```python
from build123d import *

# Parameters (mm, degrees)
F0_W      = 1120
F0_H      = 722
F1_DEPTH  = 40
F2_W      = 70
F2_H      = 725
F3_DEPTH  = 10
F5_D      = 30
F7_D      = 30
F8_W      = 70
F8_H      = 725
F9_DEPTH  = 10
F11_D     = 30
F12_W     = 1060
F12_H     = 680
F13_DEPTH = 40.001


with BuildPart() as f1:
    # F0 (on Front) → F1 (new body)
    with BuildSketch(Plane.XZ):
        Rectangle(F0_W, F0_H)
    extrude(amount=F1_DEPTH)

    # F2 (on Front) → F3 (join)
    with BuildSketch(Plane.XZ):
        with Locations((590, 0)):
            Rectangle(F2_W, F2_H)
    extrude(amount=F3_DEPTH)

    # F5 (through all)
    with Locations(Plane.XZ.offset(10)):
        with Locations((585, 142.5)):
            Hole(F5_D / 2)

    # F7 (through all)
    with Locations(Plane.XZ.offset(10)):
        with Locations((585, -142.5)):
            Hole(F7_D / 2)

    # F8 (on Front) → F9 (join)
    with BuildSketch(Plane.XZ):
        with Locations((-590, 0)):
            Rectangle(F8_W, F8_H)
    extrude(amount=F9_DEPTH)

    # F11 (through all)
    with Locations(Plane.XZ.offset(10)):
        with Locations((-585, 142.5), (-585, -142.556826)):
            Hole(F11_D / 2)

    # F12 (on face) → F13 (cut, through all)
    with BuildSketch(Plane.XZ.offset(40)):
        Rectangle(F12_W, F12_H)
    extrude(amount=-F13_DEPTH, mode=Mode.SUBTRACT)


solid = f1.part
```
Work out the finished part from the listing and answer in its coordinate system (mm). A direction names the side the tool comes from. Give positions to 0.01 mm unless a question says otherwise; leave off trailing zeros. Order: outer loops, then holes, each group sorted by start corner. A loop starts at its lowest first (then second) coordinate and runs counter-clockwise, first axis right, second up. Notation, with made-up numbers: (45, 45) -> (85, 45) arc R21 ccw to (85, 77) -> close; hole circle Ø6 at (31, 19). An arc over 180 degrees is marked (long way). Answer as CSV lines item,"result". Start each with the question number.
(1) Section D-D, the plane y = -27 is taken. Write down the section's boundary in (x, z).
(2) For a pull along Z with two mould halves and no side action, classify faces 4 (the flat face through (560, -25, -5)), 5 (the cylindrical face through (596.9, -4.93, 133.37)), 6 (the flat face through (-7, -20, -340)) as released by +Z, released by -Z, zero draft, split by the parting line, or undercut.
(3) Each of these flat-tipped pins is pushed along its axis until it touches: pin 1 Ø1.5 at (x, y) = (293.5, -9) entering from +Z; pin 2 Ø20 at (x, y) = (41.5, -10.5) entering from -Z; pin 3 Ø18 at (x, z) = (-585, 142.5) entering from -Y; pin 4 Ø8 at (y, z) = (-30.5, -220) entering from -X. Where does it stop, or does it pass through?
(4) Section C-C, the plane x = 585 is taken. Write down the section's boundary in (y, z), plus the area to 3 significant figures.
(5) Consider line 1 along Z through (x, y) = (585, -3.25); line 2 along X through (y, z) = (-31.5, 123); line 3 along Z through (x, y) = (-585, -2). Determine where each line is inside the solid, lowest interval first.
(6) Section A-A, the plane z = -276.5 is taken. Write down the section's boundary in (x, y).
(7) Which of the six approach directions +Z, -Z, +X, -X, +Y, -Y give full straight-line access (tool end or side, diameter ignored) to faces 1 (the flat face through (-560, -25, -5)), 2 (the flat face through (-7, -20, 340)), 3 (the flat face through (-3, 0, 351))?
(8) Section B-B, the plane z = 142.5 is taken. Write down the section's boundary in (x, y).
Entries:
1,outline,"(-560, -361) -> (560, -361) -> (560, 361) -> (-560, 361) -> close; hole (-530, -340) -> (530, -340) -> (530, 340) -> (-530, 340) -> close"
2,face 4,"zero draft"
2,face 5,"undercut"
2,face 6,"undercut"
3,pin 1,"z = 361"
3,pin 2,"z = -361"
3,pin 3,"through"
3,pin 4,"x = -560"
4,outline,"(-10, -362.5) -> (0, -362.5) -> (0, -157.5) -> (-10, -157.5) -> close; (-10, -127.5) -> (0, -127.5) -> (0, 127.5) -> (-10, 127.5) -> close; (-10, 157.5) -> (0, 157.5) -> (0, 362.5) -> (-10, 362.5) -> close"
4,area,"6,650 mm²"
5,line 1,"-362.5 to -157.5, -127.5 to 127.5, 157.5 to 362.5"
5,line 2,"-560 to -530, 530 to 560"
5,line 3,"-362.5 to -157.56, -127.56 to 127.5, 157.5 to 362.5"
6,outline,"(-625, -10) -> (-560, -10) -> (-560, -40) -> (-530, -40) -> (-530, 0) -> (-625, 0) -> close; (530, -40) -> (560, -40) -> (560, -10) -> (625, -10) -> (625, 0) -> (530, 0) -> close"
7,face 1,"+Z, -Z, -X, -Y"
7,face 2,"+Y, -Y"
7,face 3,"+Z, -Z, +X, -X, +Y"
8,outline,"(-625, -10) -> (-600, -10) -> (-600, 0) -> (-625, 0) -> close; (-570, -10) -> (-560, -10) -> (-560, -40) -> (-530, -40) -> (-530, 0) -> (-570, 0) -> close; (530, -40) -> (560, -40) -> (560, -10) -> (570, -10) -> (570, 0) -> (530, 0) -> close; (600, -10) -> (625, -10) -> (625, 0) -> (600, 0) -> close"
